Here's how the part is built. I have some questions about the finished solid (model axes, mm). A direction names the side the tool comes from. Coordinates: 2 decimals unless noted, no trailing zeros. Order: outer loops, then holes, each group sorted by start corner. A loop starts at its lowest first (then second) coordinate and runs counter-clockwise, first axis right, second up. Notation, with made-up numbers: (-20.5, 86) - (15.5, 86) arc R12 ccw to (15.5, 91) - close; hole circle Ø2 at (88, -37.5). An arc over 180 degrees is marked (long way). Answer in a Markdown table with one row per item. Add a question column.
Item 1: I want a section at A-A (z = 1.9). Count the separate pieces of the cut face and the enclosed holes in it, plus the area to 3 significant figures.
Item 2: I want a section at B-B (y = -64). Please give me the cut outline in (x, z).
Item 3: On a 3-axis mill with a long thin cutter (end or side, diameter ignored), from which of +Z, -Z, +X, -X, +Y, -Y can I reach the whole of each face in a straight line? I mean faces 4 (the flat face through (37, 86, 2)), 5 (the flat face through (-31.056, 76.542, 1.726)), 6 (the cylindrical face through (25.37, 52.18, 1.77)). Say none if no direction works.
Item 4: Thinking about a two-plate mould opening in Y: for faces 1 (the flat face through (-1, 5, 3.5)), 2 (the cylindrical face through (-25.513, 71.707, 1.774)), 3 (the cylindrical face through (44.63, 31.82, 1.77)), which applies, +Y half, -Y half, draft (parallel to the pull), parting line (faces both ways), or undercut?
Item 5: I want a section at C-C (y = -38.5). Please give me the cut outline in (x, z).
Item 6: If I drill on line 1 along X through (y, z) = (-2, 2.6); line 2 along X through (y, z) = (-73.5, 2.3); line 3 along Y through (x, z) = (1, 3.25), over which ranges is the centre line in solid material (lowest first)? Write a range as from..to.
Item 7: Will these pins go through, and if not, where does the flat tip stop? pin 1 Ø2 at (x, y) = (32, 86) entering from -Z; pin 2 Ø1.5 at (x, z) = (26.5, 2.5) entering from -Y; pin 3 Ø1.8 at (y, z) = (64, 2) entering from +X; pin 4 Ø10 at (x, y) = (-23.5, 19.5) entering from -Z.
```python
from build123d import *

# Parameters (mm, degrees)
F0_R     = 1.5
F0_W     = 2.5
F0_H     = 22
F0_R_2   = 1.375
F1_DEPTH = 3.5
F2_R     = 5


# Not quite as in the source:
# - a feature names something its author has since deleted; it is built from what else it names


with BuildPart() as f1:
    # F0 (on Top) → F1 (new body)
    with BuildSketch(Plane.XY):
        with BuildLine():
            Line((-25, 52), (-45, 32))
            Line((-45, 32), (-45, -28))
            Line((-45, -28), (-25, -48))
            Line((-25, -48), (-25, -88))
            ThreePointArc((-25, -88), (-23.5355339059, -91.5355339059), (-20, -93))
            Line((-20, -93), (20, -93))
            ThreePointArc((20, -93), (23.5355339059, -91.5355339059), (25, -88))
            Line((25, -88), (25, -48))
            Line((25, -48), (45, -28))
            Line((45, -28), (45, 32))
            Line((45, 32), (25, 52))
            Line((25, 52), (25, 72))
            Line((25, 72), (37, 81))
            Line((37, 81), (37, 91))
            Line((37, 91), (25, 100))
            Line((25, 100), (-25, 100))
            Line((-25, 100), (-37, 91))
            Line((-37, 91), (-37, 81))
            Line((-37, 81), (-25, 72))
            Line((-25, 72), (-25, 52))
        make_face()
        with Locations((-20, -88)):
            Circle(F0_R, mode=Mode.SUBTRACT)
        with Locations((-8.5, -73.5)):
            Circle(F0_R, mode=Mode.SUBTRACT)
        with Locations((-40, -18)):
            Circle(F0_R, mode=Mode.SUBTRACT)
        with Locations((-40, 2)):
            Circle(F0_R, mode=Mode.SUBTRACT)
        with Locations((-33.75, 0)):
            Rectangle(F0_W, F0_H, mode=Mode.SUBTRACT)
        with Locations((-8.5, -34.5)):
            Circle(F0_R, mode=Mode.SUBTRACT)
        with Locations((0, -88)):
            Circle(F0_R, mode=Mode.SUBTRACT)
        with Locations((8, -73.5)):
            Circle(F0_R, mode=Mode.SUBTRACT)
        with Locations((20, -88)):
            Circle(F0_R, mode=Mode.SUBTRACT)
        with Locations((19, -34.5)):
            Circle(F0_R, mode=Mode.SUBTRACT)
        with Locations((20, -26.5)):
            Circle(F0_R, mode=Mode.SUBTRACT)
        with Locations((3.25, 0)):
            Rectangle(F0_W, F0_H, mode=Mode.SUBTRACT)
        with Locations((40, -18)):
            Circle(F0_R, mode=Mode.SUBTRACT)
        with Locations((40, 2)):
            Circle(F0_R, mode=Mode.SUBTRACT)
        with Locations((-40, 22)):
            Circle(F0_R, mode=Mode.SUBTRACT)
        with Locations((-21.5, 40)):
            Circle(F0_R, mode=Mode.SUBTRACT)
        with Locations((-32, 86)):
            Circle(F0_R_2, mode=Mode.SUBTRACT)
        with Locations((-20, 95)):
            Circle(F0_R, mode=Mode.SUBTRACT)
        with Locations((20, 16.5)):
            Circle(F0_R, mode=Mode.SUBTRACT)
        with Locations((21.5, 40)):
            Circle(F0_R, mode=Mode.SUBTRACT)
        with Locations((40, 22)):
            Circle(F0_R, mode=Mode.SUBTRACT)
        with Locations((0, 95)):
            Circle(F0_R, mode=Mode.SUBTRACT)
        with Locations((20, 95)):
            Circle(F0_R, mode=Mode.SUBTRACT)
        with Locations((32, 86)):
            Circle(F0_R_2, mode=Mode.SUBTRACT)
    extrude(amount=F1_DEPTH)

    # F2
    f2_edges = [f1.edges().sort_by_distance(p)[0] for p in [
        (-45, -28, 1.75),
        (-25, -48, 1.75),
        (25, -48, 1.75),
        (45, -28, 1.75),
        (45, 32, 1.75),
        (25, 52, 1.75),
        (25, 72, 1.75),
        (-25, 52, 1.75),
        (-45, 32, 1.75),
        (-25, 72, 1.75),
        (-37, 81, 1.75),
        (-37, 91, 1.75),
        (-25, 100, 1.75),
        (25, 100, 1.75),
        (37, 91, 1.75),
        (37, 81, 1.75),
    ]]
    fillet(f2_edges, radius=F2_R)


solid = f1.part
```
Values follow:
| question | item | result |
|---|---|---|
| 1 | separate pieces | 1 |
| 1 | enclosed holes | 24 |
| 1 | area | 13,000 mm^2 |
| 2 | outline | (-25, 0) - (25, 0) - (25, 3.5) - (-25, 3.5) - close |
| 3 | face 4 | +Z, -Z, +X, +Y |
| 3 | face 5 | +Z, -Z, -X |
| 3 | face 6 | +Z, -Z, +X |
| 4 | face 1 | draft |
| 4 | face 2 | undercut |
| 4 | face 3 | +Y half |
| 5 | outline | (-34.5, 0) - (34.5, 0) - (34.5, 3.5) - (-34.5, 3.5) - close |
| 6 | line 1 | x = -45..-35, -32.5..2, 4.5..45 |
| 6 | line 2 | x = -25..-10, -7..6.5, 9.5..25 |
| 6 | line 3 | y = -93..-89.12, -86.88..93.88, 96.12..100 |
| 7 | pin 1 | passes through |
| 7 | pin 2 | stops at y = -47.44 |
| 7 | pin 3 | stops at x = 25 |
| 7 | pin 4 | stops at z = 0 |
